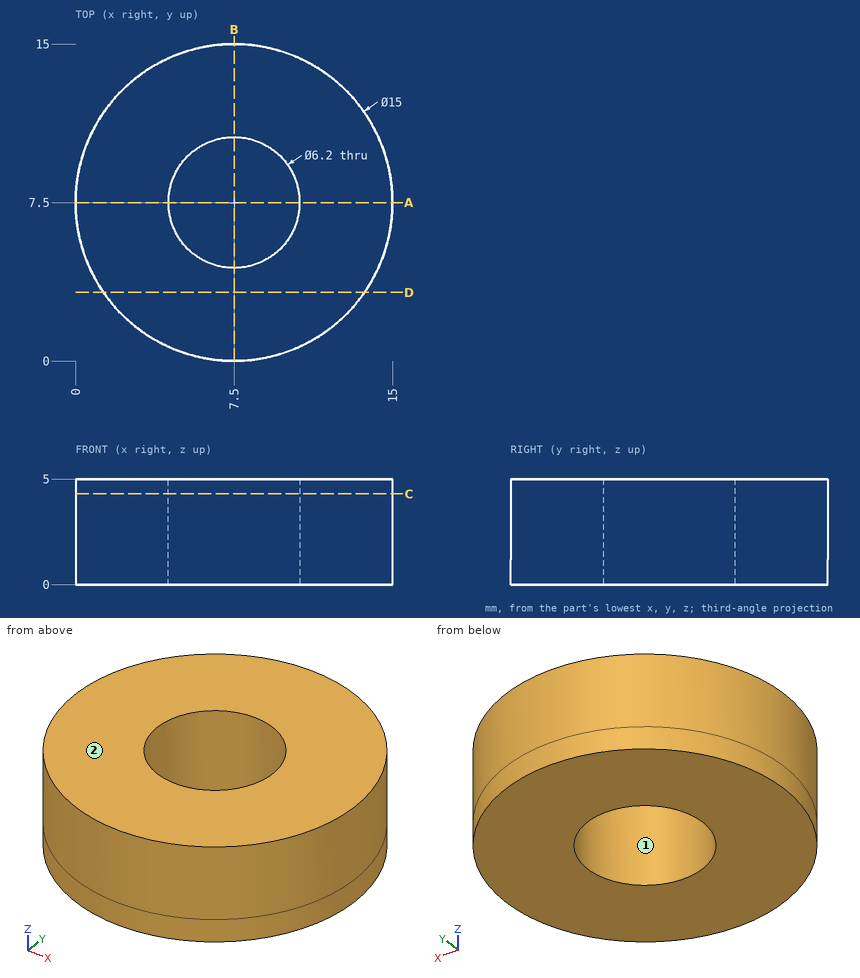
Input: dimensioned drawing with shaded views. Units: mm. Origin: part minimum x, y, z. Coordinates: 2 decimals unless noted, no trailing zeros. Order: outer loops, then holes, each group sorted by start corner. A loop starts at its lowest first (then second) coordinate and runs counter-clockwise, first axis right, second up. Notation, with made-up numbers: (36, -26.75) - (54, -26.75) arc R29 cw to (54, 0.25) - close; hole circle Ø6 at (45, -16). An arc over 180 degrees is marked (long way). Return JSON: item names as keys, results as strings. Group by question number.
1. Cut plane D-D (y = 3.25). Output: boundary loops of the cut face in (x, z), plus the area to 3 significant figures.
2. Cut plane A-A (y = 7.5). Output: boundary loops of the cut face in (x, z).
3. Cut plane C-C (z = 4.3). Output: boundary loops of the cut face in (x, y).
4. Pull-direction query (Y, two-part tool) for the marked faces 1 and 2; classes: pulls with the +Y half, pulls with the -Y half, needs draft (parallel to the pull), parting line crosses it, or undercut.
5. Material intervals for line 1 along Y through (x, z) = (7.5, 1.35); line 2 along X through (y, z) = (10.25, 3.6); line 3 along Y through (x, z) = (6.25, 0.55), sorted ascending. Write a range as [from, to].
6. Pin query (flat end, axial travel): pin 1 (2 mm diameter, centred on y = 13.5, z = 1, fed in from -X); pin 2 (8 mm diameter, centred on x = 7, y = 8.5, fed in from +Z); pin 3 (5.5 mm diameter, centred on x = 7.5, y = 7.5, fed in from -Z). Return the tip coordinate at first contact, or that it passes through.
Resolved:
{
 "1": {"outline": "(1.32, 0) - (13.68, 0) - (13.68, 5) - (1.32, 5) - close", "area": "61.8 mm²"},
 "2": {"outline": "(0, 0) - (4.4, 0) - (4.4, 5) - (0, 5) - close; (10.6, 0) - (15, 0) - (15, 5) - (10.6, 5) - close"},
 "3": {"outline": "circle Ø15 at (7.5, 7.5); hole circle Ø6.2 at (7.5, 7.5)"},
 "4": {"face 1": "undercut", "face 2": "needs draft"},
 "5": {"line 1": "y = [0, 4.4], [10.6, 15]", "line 2": "x = [0.52, 6.07], [8.93, 14.48]", "line 3": "y = [0.1, 4.66], [10.34, 14.9]"},
 "6": {"pin 1": "stops at x = 1.91", "pin 2": "stops at z = 5", "pin 3": "passes through"}
}
